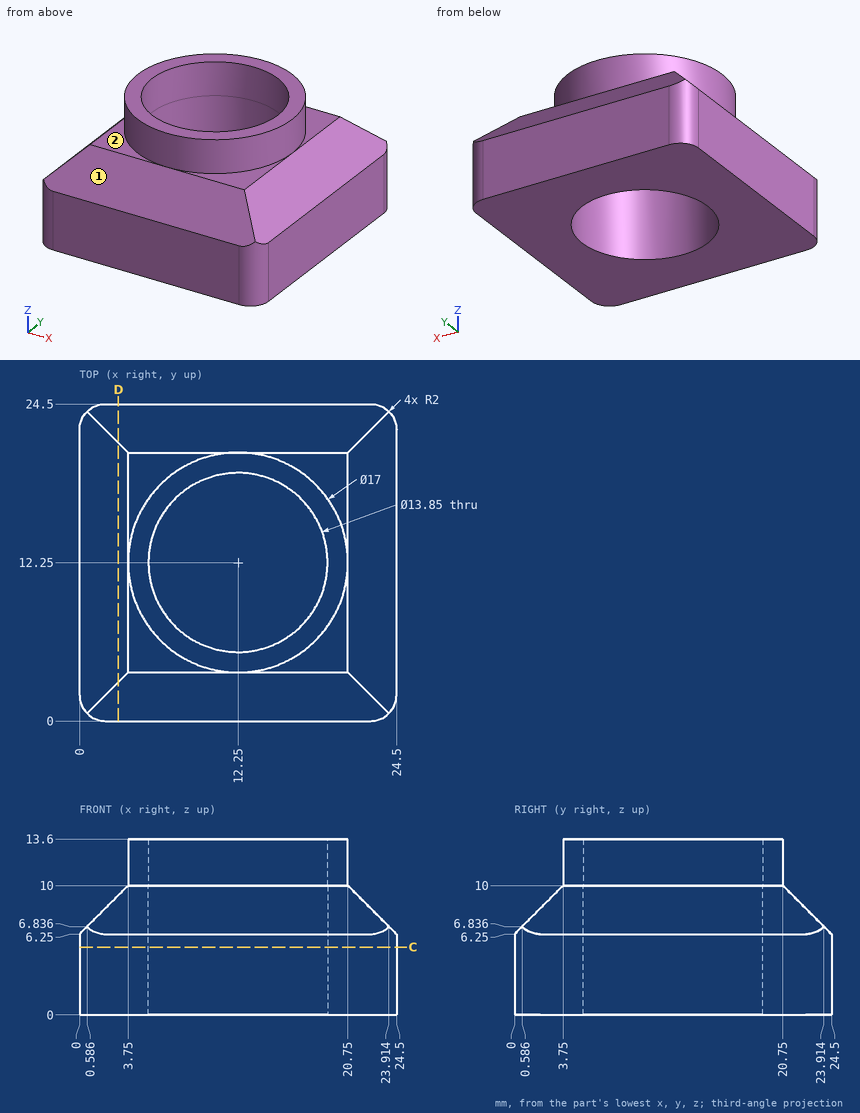
Design review of the part shown in the three views and the two pictorial views. Dimensions are in mm from the part's minimum x, y and z. A direction names the side the tool comes from. Give positions to 0.01 mm unless a question says otherwise; leave off trailing zeros. Loops run counter-clockwise (first coordinate to the right, second up) from the corner with the lowest first, then second, coordinate; pieces in that order, holes last. Notation, with made-up numbers: (-23, 82.5) -> (36, 82.5) arc R13 ccw to (36, 88.5) -> close; hole circle Ø5 at (80, -4). An arc over 180 degrees is marked (long way). One line per item, written item: value.
Q1. We need section D-D on x = 3. Give the boundary of the cut face in (y, z).
Numbers:
outline: (0, 0) -> (24.5, 0) -> (24.5, 6.25) -> (21.5, 9.25) -> (3, 9.25) -> (0, 6.25) -> close
Q2. For pin 1 Ø6 at (y, z) = (10.5, 10.5) entering from -X; pin 2 Ø1.5 at (x, z) = (12, 9) entering from +Y, all flat-tipped, find the tip position at first contact; note any pin that passes through.
Numbers:
pin 1: stops at x = 1.25
pin 2: stops at y = 22.5
Q3. For L1, parallel to Y at x = 12.25, z = 12.35 (3 decimals); L2, parallel to Y at x = 12.25, z = 2 (3 decimals); L3, parallel to Z at x = 16, y = 4, list the stretches that pass through material, from the lowest coordinate up.
Numbers:
L1: y = 3.75 to 5.325, 19.175 to 20.75
L2: y = 0 to 5.325, 19.175 to 24.5
L3: z = 0 to 10
Q4. We need section C-C on z = 5.25. Give the boundary of the cut face in (x, y) (3 decimals).
Numbers:
outline: (0, 2) arc R2 ccw to (2, 0) -> (22.5, 0) arc R2 ccw to (24.5, 2) -> (24.5, 22.5) arc R2 ccw to (22.5, 24.5) -> (2, 24.5) arc R2 ccw to (0, 22.5) -> close; hole circle Ø13.85 at (12.25, 12.25)
Q5. Machinability: for the marked faces 1 and 2, which of the approach directions +Z, -Z, +X, -X, +Y, -Y give a long, thin tool a straight path to every point of the face, cutting with its end or side? Answer none if there is none.
Numbers:
face 1: +Z, +X, -X, -Y
face 2: +Z
